Input: part model. Units: mm. Frame: model coordinates. Face numbers are marked on the shaded views. A direction names the side the tool comes from. Coordinates: 2 decimals unless noted, no trailing zeros. Order: outer loops, then holes, each group sorted by start corner. A loop starts at its lowest first (then second) coordinate and runs counter-clockwise, first axis right, second up. Notation, with made-up numbers: (27.25, 63.25) -> (50.25, 63.25) arc R25 cw to (50.25, 89.25) -> close; hole circle Ø2 at (82, -34.5). An arc over 180 degrees is marked (long way). One line per question, with ' | ' between items.
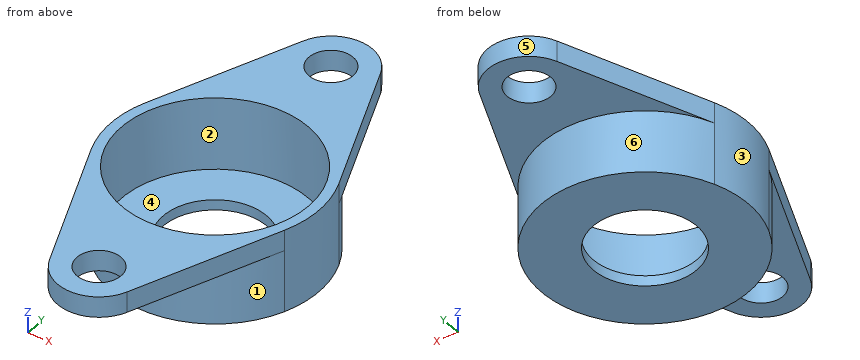
Autodesk Inventor part; units mm, degrees
ref_plane "YZ Plane" through (0, 0, 0) normal (1, 0, 0) x (0, 1, 0)
ref_plane "XZ Plane" through (0, 0, 0) normal (0, 1, 0) x (-1, 0, 0)
ref_plane "XY Plane" through (0, 0, 0) normal (0, 0, 1) x (1, 0, 0)
sketch "Sketch1" plane through (0, 0, 0) normal (0, 0, 1) x (1, 0, 0)
  circle A0 centre (0, 0) radius 14.2875 construction
  line L0 (-22.225, 0) -> (22.225, 0)
  line L1 (0, -44.45) -> (0, 44.45)
  arc A1 (5.8866, 27.7812) -> (-5.8866, 27.7812) centre (0, 25.4) ccw
  arc A2 (-5.8866, -27.7812) -> (5.8866, -27.7812) centre (0, -25.4) ccw
  line L2 (5.8866, -27.7812) -> (14.7165, -5.9531)
  line L3 (-5.8866, -27.7812) -> (-14.7165, -5.9531)
  line L4 (-5.8866, 27.7812) -> (-14.7165, 5.9531)
  line L5 (5.8866, 27.7812) -> (14.7165, 5.9531)
  arc A3 (-14.7165, 5.9531) -> (-14.7165, -5.9531) centre (0, 0) ccw
  arc A4 (14.7165, -5.9531) -> (14.7165, 5.9531) centre (0, 0) ccw
  circle A5 centre (0, 0) radius 7.9375
  dimension "d1" = 28.575
  dimension "d2" = 15.875
  dimension "d3" = 15.875
  dimension "d4" = 6.35
  dimension "d5" = 25.4
  dimension "d6" = 25.4
  dimension "d7" = 15.875
extrude "Extrusion1" add sketch "Sketch1" against normal blind 12.7 contours A3 L4 A1 L1 A5 L0 | L0 A5 L1 A2 L3 A3 | L1 A1 L5 A4 L0 A5 | A5 L0 A4 L2 A2 L1
sketch "Sketch2" plane through (0, 0, -12.7) normal (0, 0, -1) x (-1, 0, 0)
  line L0 (-5.8866, -27.7812) -> (-14.7165, -5.9531)
  arc A0 (-5.8866, -27.7812) -> (5.8866, -27.7812) centre (0, -25.4) ccw
  line L1 (14.7165, -5.9531) -> (5.8866, -27.7812)
  arc A1 (14.7165, -5.9531) -> (14.7165, 5.9531) centre (0, 0) ccw
  line L2 (5.8866, 27.7812) -> (14.7165, 5.9531)
  arc A2 (5.8866, 27.7812) -> (-5.8866, 27.7812) centre (0, 25.4) ccw
  line L3 (-14.7165, 5.9531) -> (-5.8866, 27.7812)
  arc A3 (-14.7165, 5.9531) -> (-14.7165, -5.9531) centre (0, 0) ccw
  circle A4 centre (0, 0) radius 15.875
extrude "Extrusion2" cut sketch "Sketch2" against normal blind 9.525 contours L0 A4 L1 A0 | L3 A2 L2 A4
sketch "Sketch3" plane through (0, 0, 0) normal (0, 0, 1) x (1, 0, 0)
  circle A0 centre (0, 0) radius 7.9375
  arc A1 (-14.7165, 5.9531) -> (-14.7165, -5.9531) centre (0, 0) ccw
  circle A2 centre (0, 0) radius 14.3129
  dimension "d12" = 28.6258
extrude "Extrusion3" cut sketch "Sketch3" against normal blind 11.1125
sketch "Sketch4" plane through (0, 0, 0) normal (0, 0, 1) x (1, 0, 0)
  arc A0 (-5.8866, -27.7812) -> (5.8866, -27.7812) centre (0, -25.4) ccw
  arc A1 (5.8866, 27.7812) -> (-5.8866, 27.7812) centre (0, 25.4) ccw
hole "Hole1" at (0, 25.4, 0) at (0, -25.4, 0) direction (0, 0, -1) diameter 6.7564 end through all
properties part number "bearing block wheel mount"
1. Mould query, pull axis X, two halves, no side actions, for the marked faces 1, 2 and 3. Classes: released by +X, released by -X, zero draft, split by the parting line, or undercut.
Recorded:
face 1: split by the parting line | face 2: undercut | face 3: released by -X
2. Access query for the marked faces 4, 5 and 6. Directions: +Z, -Z, +X, -X, +Y, -Y. A direction counts if a zero-diameter tool reaches every point of the face in a straight line with its end or side. Return the directions, or none.
Recorded:
face 4: +Z | face 5: +Z, -Z, +Y | face 6: -Z, +Y
3. Ray query, line 1 (Y direction, x = -3, z = -2.5); line 2 (Y direction, x = 12.5, z = -0.75); line 3 (X direction, y = -25.4, z = -0.75). Return the intervals inside material, ascending. Write a range as [from, to].
Recorded:
line 1: y = [-31, -26.95], [-23.85, -13.99], [13.99, 23.85], [26.95, 31] | line 2: y = [-11.43, -6.97], [6.97, 11.43] | line 3: x = [-6.85, -3.38], [3.38, 6.85]
4. Cut plane C-C, the plane x = 7. Return loops of the section in (y, z) (1 decimal).
Recorded:
outline: (-25, -3.2) -> (-14.2, -3.2) -> (-14.2, -12.7) -> (-3.7, -12.7) -> (-3.7, -11.1) -> (-12.5, -11.1) -> (-12.5, 0) -> (-25, 0) -> close; (3.7, -12.7) -> (14.2, -12.7) -> (14.2, -3.2) -> (25, -3.2) -> (25, 0) -> (12.5, 0) -> (12.5, -11.1) -> (3.7, -11.1) -> close
5. Cut plane D-D, the plane y = -23. Return loops of the section in (x, z) (3 decimals), and give its area (3 significant figures).
Recorded:
outline: (-7.821, -3.175) -> (-2.377, -3.175) -> (-2.377, 0) -> (-7.821, 0) -> close; (2.377, -3.175) -> (7.821, -3.175) -> (7.821, 0) -> (2.377, 0) -> close | area: 34.6 mm^2
6. Cut plane B-B, the plane y = 0. Return loops of the section in (x, z).
Recorded:
outline: (-15.87, -12.7) -> (-7.94, -12.7) -> (-7.94, -11.11) -> (-14.31, -11.11) -> (-14.31, 0) -> (-15.87, 0) -> close; (7.94, -12.7) -> (15.87, -12.7) -> (15.87, 0) -> (14.31, 0) -> (14.31, -11.11) -> (7.94, -11.11) -> close
7. Cut plane A-A, the plane x = 0. Return loops of the section in (y, z) (1 decimal).
Recorded:
outline: (-31.7, -3.2) -> (-28.8, -3.2) -> (-28.8, 0) -> (-31.7, 0) -> close; (-22, -3.2) -> (-15.9, -3.2) -> (-15.9, -12.7) -> (-7.9, -12.7) -> (-7.9, -11.1) -> (-14.3, -11.1) -> (-14.3, 0) -> (-22, 0) -> close; (7.9, -12.7) -> (15.9, -12.7) -> (15.9, -3.2) -> (22, -3.2) -> (22, 0) -> (14.3, 0) -> (14.3, -11.1) -> (7.9, -11.1) -> close; (28.8, -3.2) -> (31.7, -3.2) -> (31.7, 0) -> (28.8, 0) -> close
8. Pin query (flat end, axial travel): pin 1 Ø1.5 at (y, z) = (-18.5, -5) entering from -X; pin 2 Ø9 at (x, y) = (0, -25.4) entering from -Z (3 decimals); pin 3 Ø4 at (y, z) = (14.5, -10) entering from +X; pin 4 Ø4 at (x, y) = (7.5, -8.5) entering from +Z. Return the tip coordinate at first contact, or that it passes through.
Recorded:
pin 1: passes through | pin 2: stops at z = -3.175 | pin 3: stops at x = 9.79 | pin 4: stops at z = -11.11
